Input: part model. Units: mm. Frame: model coordinates. A direction names the side the tool comes from. Give positions to 0.01 mm unless a question says otherwise; leave off trailing zeros. Loops run counter-clockwise (first coordinate to the right, second up) from the corner with the lowest first, then second, coordinate; pieces in that order, holes last. Notation, with made-up numbers: M -21.5,13 L 19.5,13 A27 cw 19.5,35 Z; hole C -37,-19 d11. An arc over 180 degrees is marked long. Answer as a JSON object with one key per item and string values. Group by question number.
1) First-contact query: P1, Ø3, axis at y = 31.5, z = 20, coming from the -X side; P2, Ø6, axis at y = -27, z = 6, coming from the +X side; P3, Ø5.5, axis at y = 85, z = 9.5, coming from the +X side; P4, Ø7.5, axis at y = 76.2, z = 12.065, coming from the +X side. Flat tips, straight axial feed; report the tip coordinate or a pass-through.
2) Section query A-A on x = -38.5. Return loops of the section in (y, z) (3 decimals).
3) Section query B-B on y = 0. Return loops of the section in (x, z), plus the area to 3 significant figures.
4) Ray query, L1, parallel to Z at x = -127.25, y = 76.2; L2, parallel to Y at x = -54.5, z = 12; L3, parallel to Y at x = -131, z = 12.75. Return the intervals inside material, ascending.
5) Draft query along Z for faces 4 (the flat face through (-146, -76.2, 12)), 5 (the flat face through (-53, -19, 24.13)), 6 (the cylindrical face through (-127.472, 71.478, 12.685)). Return one class per face: +Z half, -Z half, draft (parallel to the pull), parting line (faces both ways), or undercut.
6) Section query C-C on x = 0. Return loops of the section in (y, z).
7) Access query for faces 1 (the flat face through (-58.38, -83.07, 11.9)), 2 (the flat face through (-127, 38.1, 12)), 3 (the flat face through (-99.9, -50.64, 11.9)). Directions: +Z, -Z, +X, -X, +Y, -Y. A direction counts if a zero-diameter tool reaches every point of the face in a straight line with its end or side. Return the directions, or none.
from build123d import *

# Parameters (mm, degrees)
SKETCH1_R           = 50.8
BOSS_EXTRUDE1_DEPTH = 24.13
FILLET1_R           = 10.16
SKETCH2_R           = 4.7625
CUT_EXTRUDE1_DEPTH  = 252.642736633


with BuildPart() as part:
    # Sketch1 → Boss-Extrude1 (new body)
    with BuildSketch(Plane.XY):
        with BuildLine():
            Line((-133.35, 88.9), (-133.35, 38.1))
            Line((-133.35, 38.1), (-120.65, 38.1))
            Line((-120.65, 38.1), (-100.755098441, 28.715816927))
            ThreePointArc((-100.755098441, 28.715816927), (-83.188973521, 6.337707108), (-90.601125221, -21.128791593))
            Line((-90.601125221, -21.128791593), (-139.7, -76.2))
            Line((-139.7, -76.2), (-152.4, -76.2))
            Line((-152.4, -76.2), (-152.4, -127))
            Line((-152.4, -127), (-139.7, -127))
            Line((-139.7, -127), (-139.7, -106.68))
            Line((-139.7, -106.68), (17.704429235, -60.981990665))
            ThreePointArc((17.704429235, -60.981990665), (63.039807772, 7.631031129), (2.642419241, 63.444996813))
            Line((2.642419241, 63.444996813), (-120.65, 68.58))
            Line((-120.65, 68.58), (-120.65, 88.9))
            Line((-120.65, 88.9), (-133.35, 88.9))
        make_face()
        with Locations(Location((0, 0, 0), (0, 0, 180))):
            Circle(SKETCH1_R, mode=Mode.SUBTRACT)
        with BuildLine():
            Line((-46.037431664, 52.76145265), (-110.49514893, 55.446050662))
            ThreePointArc((-110.49514893, 55.446050662), (-114.353417179, 52.549377789), (-112.279082271, 48.193452823))
            Line((-112.279082271, 48.193452823), (-70.985594525, 28.715816927))
            ThreePointArc((-70.985594525, 28.715816927), (-67.368742902, 26.71210826), (-64.042949916, 24.25536955))
            ThreePointArc((-64.042949916, 24.25536955), (-60.727043781, 23.453741785), (-58.09853243, 25.628314996))
            ThreePointArc((-58.09853243, 25.628314996), (-51.868282156, 36.632380569), (-43.581110206, 46.183729096))
            ThreePointArc((-43.581110206, 46.183729096), (-42.626724096, 50.287620053), (-46.037431664, 52.76145265))
        make_face(mode=Mode.SUBTRACT)
        with BuildLine():
            Line((-77.6210071, -25.653934719), (-122.808045193, -76.337474888))
            ThreePointArc((-122.808045193, -76.337474888), (-123.43951378, -83.950303149), (-116.297827314, -86.661432273))
            Line((-116.297827314, -86.661432273), (-32.118533433, -62.222309585))
            ThreePointArc((-32.118533433, -62.222309585), (-29.396609186, -59.006115837), (-31.302640742, -55.248481269))
            ThreePointArc((-31.302640742, -55.248481269), (-46.04089289, -43.731981225), (-56.784547657, -28.421209464))
            ThreePointArc((-56.784547657, -28.421209464), (-66.469460728, -21.515994345), (-77.6210071, -25.653934719))
        make_face(mode=Mode.SUBTRACT)
    extrude(amount=BOSS_EXTRUDE1_DEPTH)

    # Fillet1
    fillet1_edges = [part.edges().sort_by_distance(p)[0] for p in [
        (-120.65, 68.58, 12.065),
        (-139.7, -106.68, 12.065),
    ]]
    fillet(fillet1_edges, radius=FILLET1_R)

    # Sketch2 → Cut-Extrude1 (cut, through all)
    with BuildSketch(Plane.ZY.offset(152.4)):
        with Locations(Location((12.065, -114.3, 0), (0, 0, 270))):
            Circle(SKETCH2_R)
        with Locations(Location((12.065, 76.2, 0), (0, 0, 180))):
            Circle(SKETCH2_R)
    extrude(amount=-CUT_EXTRUDE1_DEPTH, mode=Mode.SUBTRACT)


solid = part.part
Output:
{
 "1": {"P1": "stops at x = -109.84", "P2": "stops at x = 58.79", "P3": "stops at x = -120.65", "P4": "passes through"},
 "2": {"outline": "M -77.299,0 L -64.075,0 L -64.075,24.13 L -77.299,24.13 Z; M -50.498,0 L -33.142,0 L -33.142,24.13 L -50.498,24.13 Z; M 33.142,0 L 65.159,0 L 65.159,24.13 L 33.142,24.13 Z"},
 "3": {"outline": "M -82.55,0 L -50.8,0 L -50.8,24.13 L -82.55,24.13 Z; M 50.8,0 L 63.5,0 L 63.5,24.13 L 50.8,24.13 Z", "area": "1,070 mm^2"},
 "4": {"L1": "z = 0 to 7.3, 16.83 to 24.13", "L2": "y = -81.94 to -68.72, -32.59 to 32.59, 53.11 to 65.82", "L3": "y = -104.15 to -66.44, 38.1 to 71.49, 80.91 to 88.9"},
 "5": {"face 4": "draft", "face 5": "+Z half", "face 6": "undercut"},
 "6": {"outline": "M -66.12,0 L -50.8,0 L -50.8,24.13 L -66.12,24.13 Z; M 50.8,0 L 63.56,0 L 63.56,24.13 L 50.8,24.13 Z"},
 "7": {"face 1": "+Z, -Z, +X, -Y", "face 2": "+Z, -Z, -X", "face 3": "+Z, -Z"}
}
